For this review, take the finished solid that the model builds, in its own axes (mm). A direction names the side the tool comes from. Give positions to 0.01 mm unless a question says otherwise; leave off trailing zeros. Loops run counter-clockwise (first coordinate to the right, second up) from the corner with the lowest first, then second, coordinate; pieces in that order, holes last. Notation, with made-up numbers: (-36.75, 19) - (-12.75, 19) arc R6 ccw to (-12.75, 25) - close; hole circle Ø3 at (0, 82). An arc over 180 degrees is marked (long way). Answer as CSV lines item,"result".
from build123d import *

# Parameters (mm, degrees)
BOSS_EXTRUDE1_DEPTH      = 12
SKETCH4_R                = 1.5
CUT_EXTRUDE2_DEPTH       = 36.60898763
BOSS_EXTRUDE2_DEPTH      = 20
BOSS_EXTRUDE2_DEPTH_BACK = 12
SKETCH7_W                = 12
SKETCH7_H                = 12
CUT_EXTRUDE1_DEPTH       = 2
SKETCH8_W                = 6.4
SKETCH8_H                = 6.4
CUT_EXTRUDE4_DEPTH       = 47.818799643
SKETCH9_W                = 5.6
SKETCH9_H                = 3.1
CUT_EXTRUDE5_DEPTH       = 9
SKETCH10_R               = 1.7
CUT_EXTRUDE6_DEPTH       = 41.573883226
FILLET1_R                = 5


with BuildPart() as part:
    # Sketch1 → Boss-Extrude1 (new body)
    with BuildSketch(Plane.XY):
        with BuildLine():
            Line((10, 22), (10, 0))
            ThreePointArc((10, 0), (0, -10), (-10, 0))
            Line((-10, 0), (-10, 22))
            ThreePointArc((-10, 22), (0, 32), (10, 22))
        make_face()
    extrude(amount=BOSS_EXTRUDE1_DEPTH)

    # Sketch4 → Cut-Extrude2 (cut, through all)
    with BuildSketch(Plane.XY):
        Circle(SKETCH4_R)
    extrude(amount=CUT_EXTRUDE2_DEPTH, mode=Mode.SUBTRACT)

    # Sketch7 → Boss-Extrude2 (add, two sides: drawn at the far end of the back side and taken through both)
    with BuildSketch(Plane(origin=(0, 0, 0), x_dir=(0, 0, -1), z_dir=(1, 0, 0)).offset(-BOSS_EXTRUDE2_DEPTH_BACK)):
        with Locations((-6, 20)):
            Rectangle(SKETCH7_W, SKETCH7_H)
    extrude(amount=BOSS_EXTRUDE2_DEPTH + BOSS_EXTRUDE2_DEPTH_BACK)

    # Sketch2 → Cut-Extrude1 (cut)
    with BuildSketch(Plane.XY):
        with BuildLine():
            Line((-2.5, 19.73937205), (-4.37, 0.209105237))
            ThreePointArc((-4.37, 0.209105237), (-0.209105237, -4.37), (4.37, -0.209105237))
            ThreePointArc((4.37, -0.209105237), (4.375, 0), (4.37, 0.209105237))
            Line((4.37, 0.209105237), (2.5, 19.73937205))
            ThreePointArc((2.5, 19.73937205), (0, 22.01143365), (-2.5, 19.73937205))
        make_face()
    extrude(amount=CUT_EXTRUDE1_DEPTH, mode=Mode.SUBTRACT)

    # Sketch8 → Cut-Extrude4 (cut, through all)
    with BuildSketch(Plane(origin=(20, 0, 0), x_dir=(0, 0, -1), z_dir=(1, 0, 0))):
        with Locations((-6, 20)):
            Rectangle(SKETCH8_W, SKETCH8_H)
    extrude(amount=-CUT_EXTRUDE4_DEPTH, mode=Mode.SUBTRACT)

    # Sketch9 → Cut-Extrude5 (cut)
    with BuildSketch(Plane(origin=(0, 0, 0), x_dir=(-1, 0, 0), z_dir=(0, 0, -1))):
        with Locations((0, 26.25)):
            Rectangle(SKETCH9_W, SKETCH9_H)
    extrude(amount=-CUT_EXTRUDE5_DEPTH, mode=Mode.SUBTRACT)

    # Sketch10 → Cut-Extrude6 (cut, through all)
    with BuildSketch(Plane.XZ.offset(-23.2)):
        with Locations(Location((0, 6, 0), (0, 0, 270))):
            Circle(SKETCH10_R)
    extrude(amount=-CUT_EXTRUDE6_DEPTH, mode=Mode.SUBTRACT)

    # Fillet1
    # the kernel refuses this fillet: 5 mm, written as the material it adds along each edge
    with BuildSketch(Plane(origin=(10, 14, 12), x_dir=(1, 0, 0), z_dir=(0, 0, -1))) as fillet1_piece_1:
        with BuildLine():
            CenterArc((FILLET1_R, FILLET1_R), FILLET1_R, 180, 90)
            Line((0, FILLET1_R), (-FILLET1_R * 0.02, FILLET1_R))
            Line((-FILLET1_R * 0.02, FILLET1_R), (-FILLET1_R * 0.02, -FILLET1_R * 0.02))
            Line((-FILLET1_R * 0.02, -FILLET1_R * 0.02), (FILLET1_R, -FILLET1_R * 0.02))
            Line((FILLET1_R, -FILLET1_R * 0.02), (FILLET1_R, 0))
        make_face()
    extrude(amount=12)
    with BuildSketch(Plane(origin=(-9.16515139, 26, 12), x_dir=(0.5033825030764704, 0.8640636872340298, 0), z_dir=(0, 0, -1))) as fillet1_piece_2:
        with BuildLine():
            CenterArc((2.893305247, -4.966402258), FILLET1_R, 96.645859584, 53.130102354)
            Line((-1.427013189, -2.449489743), (-1.513419558, -2.399151492))
            Line((-1.513419558, -2.399151492), (-0.086406369, 0.05033825))
            Line((-0.086406369, 0.05033825), (0.011573221, 0.099328045))
            ThreePointArc((0.011573221, 0.099328045), (1.157322099, 0.032804516), (2.303070977, 0.099328045))
            Line((2.303070977, 0.099328045), (2.314644198, 0))
        make_face()
    extrude(amount=12)
    with BuildSketch(Plane(origin=(9.16515139, 26, 12), x_dir=(1, 0, 0), z_dir=(0, 0, -1))) as fillet1_piece_3:
        with BuildLine():
            CenterArc((2.83484861, -5), FILLET1_R, 90, 53.130102354)
            Line((-1.16515139, -2), (-1.24515139, -1.94))
            ThreePointArc((-1.24515139, -1.94), (-0.610920886, -0.98348678), (-0.091651514, 0.04))
            Line((-0.091651514, 0.04), (0, 0.1))
            Line((0, 0.1), (2.83484861, 0.1))
            Line((2.83484861, 0.1), (2.83484861, 0))
        make_face()
    extrude(amount=12)
    with BuildSketch(Plane(origin=(-10, 14, 0), x_dir=(-1, 0, 0), z_dir=(0, 0, 1))) as fillet1_piece_4:
        with BuildLine():
            CenterArc((5, 4), FILLET1_R, 180, 53.130102354)
            Line((0, 4), (-0.1, 4))
            Line((-0.1, 4), (-0.1, 0))
            Line((-0.1, 0), (0, -0.1))
            ThreePointArc((0, -0.1), (1, -0.1), (1.94, -0.08))
            Line((1.94, -0.08), (2, 0))
        make_face()
    extrude(amount=12)


solid = part.part
1) Consider section C-C on y = 19. Write out the cut boundary in (x, z).
From the geometry:
outline,"(-12, 0) - (-2.57, 0) - (-2.57, 2) - (2.57, 2) - (2.57, 0) - (20, 0) - (20, 2.8) - (-12, 2.8) - close; (-12, 9.2) - (20, 9.2) - (20, 12) - (-12, 12) - close"
2) Machinability: for faces 1 (the flat face through (-3.42, 10.11, 0.99)), 2 (the flat face through (4, 20, 9.2)), 3 (the cylindrical face through (-1.03, 23.94, 7.35)), 4 (the cylindrical face through (-1.5, 0.07, 6.93)), 5 (the flat face through (17, 14, 6)), which of the approach directions +Z, -Z, +X, -X, +Y, -Y give a long, thin tool a straight path to every point of the face, cutting with its end or side? Answer none if there is none.
From the geometry:
face 1,"-Z"
face 2,"+X, -X"
face 3,"+Y"
face 4,"+Z, -Z"
face 5,"+Z, -Z, +X, -Y"
3) Consider section A-A on x = 18. Write out the cut boundary in (y, z).
From the geometry:
outline,"(14, 0) - (26, 0) - (26, 12) - (14, 12) - close; hole (16.8, 2.8) - (23.2, 2.8) - (23.2, 9.2) - (16.8, 9.2) - close"
4) Consider section B-B on z = 6. Count the separate pieces of the cut face and the enclosed holes in it, and give its area (3 significant figures).
From the geometry:
separate pieces,"3"
enclosed holes,"1"
area,"662 mm^2"
5) Draft analysis for pull direction X (two halves, no side actions). For faces 6 (the flat face through (16, 26, 6)), 7 (the cylindrical face through (11, 12, 6)), 8 (the flat face through (2.8, 26, 4)), 9 (the flat face through (0, 26, 9)), state which applies: pulls with the +X half, pulls with the -X half, needs draft (parallel to the pull), parting line crosses it, or undercut.
From the geometry:
face 6,"needs draft"
face 7,"pulls with the +X half"
face 8,"undercut"
face 9,"undercut"
6) Consider section D-D on x = 0. Write out the cut boundary in (y, z) (3 decimals).
From the geometry:
outline,"(-10, 0) - (-4.375, 0) - (-4.375, 2) - (-1.5, 2) - (-1.5, 12) - (-10, 12) - close; (1.5, 2) - (22.011, 2) - (22.011, 0) - (24.7, 0) - (24.7, 4.3) - (23.2, 4.3) - (23.2, 2.8) - (16.8, 2.8) - (16.8, 9.2) - (23.2, 9.2) - (23.2, 7.7) - (24.7, 7.7) - (24.7, 9) - (27.8, 9) - (27.8, 7.7) - (32, 7.7) - (32, 12) - (1.5, 12) - close; (27.8, 0) - (32, 0) - (32, 4.3) - (27.8, 4.3) - close"
7) Insertion check: P1, Ø2.5, axis at x = 1, y = 26, coming from the -Z side; P2, Ø3, axis at x = 13, z = 2.5, coming from the +Y side; P3, Ø5.5, axis at x = 17, z = 4.5, coming from the -Y side. Each pin has a flat end and moves straight along its axis. Give the tip position at first contact, or say it passes through.
From the geometry:
P1,"stops at z = 9"
P2,"stops at y = 26.03"
P3,"stops at y = 13.94"
8) Wall thickness on line 1 (Y direction, x = 0, z = 5.25); line 2 (Y direction, x = -1, z = 7.5); line 3 (Z direction, x = 0, y = 30): over which ranges is each line inside the solid? List them lowest first. Write a range as from..to.
From the geometry:
line 1,"y = -10..-1.5, 1.5..16.8"
line 2,"y = -9.95..-1.12, 1.12..16.8, 23.2..24.7, 27.8..31.95"
line 3,"z = 0..4.3, 7.7..12"
